```python
from build123d import *

# Parameters (mm, degrees)
BOSS_EXTRUDE1_DEPTH      = 40
BOSS_EXTRUDE1_DEPTH_BACK = 40
SKETCH2_W                = 140
SKETCH2_H                = 70
CUT_EXTRUDE1_DEPTH       = 16
SKETCH3_R                = 4
CUT_EXTRUDE2_DEPTH       = 5


with BuildPart() as part:
    # Sketch1 → Boss-Extrude1 (new, two sides: drawn at the far end of the back side and taken through both)
    with BuildSketch(Plane.XY.offset(-BOSS_EXTRUDE1_DEPTH_BACK)):
        with BuildLine():
            Line((-65, 10), (65, 10))
            ThreePointArc((65, 10), (75, 0), (65, -10))
            Line((65, -10), (-65, -10))
            ThreePointArc((-65, -10), (-75, 0), (-65, 10))
        make_face()
    extrude(amount=BOSS_EXTRUDE1_DEPTH + BOSS_EXTRUDE1_DEPTH_BACK)

    # Sketch2 → Cut-Extrude1 (cut)
    with BuildSketch(Plane(origin=(0, 10, 0), x_dir=(1, 0, 0), z_dir=(0, 1, 0))):
        Rectangle(SKETCH2_W, SKETCH2_H)
    extrude(amount=-CUT_EXTRUDE1_DEPTH, mode=Mode.SUBTRACT)

    # Sketch3 → Cut-Extrude2 (cut)
    with BuildSketch(Plane.XY.offset(40)):
        with Locations((65, 0)):
            Circle(SKETCH3_R)
        with Locations((-65, 0)):
            Circle(SKETCH3_R)
        with Locations((25, 0)):
            Circle(SKETCH3_R)
    extrude(amount=-CUT_EXTRUDE2_DEPTH, mode=Mode.SUBTRACT)


solid = part.part
```
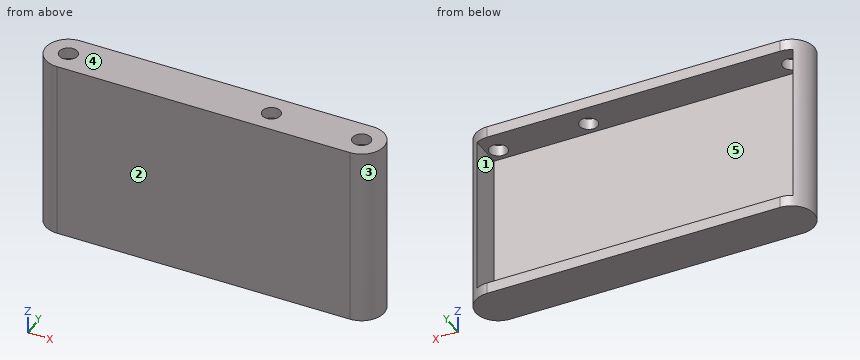
Design review of the part built by this model. Coordinates are the model's own, in mm. Face numbers are marked on the shaded views. A direction names the side the tool comes from. Give positions to 0.01 mm unless a question says otherwise; leave off trailing zeros. Order: outer loops, then holes, each group sorted by start corner. A loop starts at its lowest first (then second) coordinate and runs counter-clockwise, first axis right, second up. Notation, with made-up numbers: (67.5, -23.5) -> (121.5, -23.5) arc R23 cw to (121.5, 1.5) -> close; hole circle Ø11 at (57.5, 38.5). An arc over 180 degrees is marked (long way). Write each question's results on one line, items separated by ' | '. Start each with the question number.
Q1. Wall thickness on L1, parallel to Z at x = -44.5, y = -2.75; L2, parallel to Y at x = 25, z = 38.75; L3, parallel to Z at x = 65.5, y = -1.25: over which ranges is each line inside the solid? List them lowest first. Write a range as from..to.
Q2. Add section C-C on x = 51. Give the boundary of the cut face in (y, z), and give its area (3 significant figures).
Q3. Mouldability with a two-part tool opening along X and no side actions: class the marked faces 3, 4 and 5 as +X half, -X half, draft (parallel to the pull), parting line (faces both ways), or undercut.
Q4. Add section D-D on y = 6. Give the boundary of the cut face in (x, z), and give its area (3 significant figures).
Q5. Add section B-B on y = 0. Give the boundary of the cut face in (x, z).
Q6. For pin 1 (4.5 mm diameter, centred on y = 3.5, z = 10.5, fed in from +X); pin 2 (3 mm diameter, centred on y = 2, z = 12, fed in from +X); pin 3 (6 mm diameter, centred on x = 34, z = 24, fed in from +Y), all flat-tipped, find the tip position at first contact; note any pin that passes through.
Q7. Machinability: for the marked faces 1 and 2, which of the approach directions +Z, -Z, +X, -X, +Y, -Y give a long, thin tool a straight path to every point of the face, cutting with its end or side? Answer none if there is none.
Q8. Add section A-A on x = 25. Give the boundary of the cut face in (y, z).
Found:
1) L1: z = -40..-35, 35..40 | L2: y = -10..-4, 4..10 | L3: z = -40..-35
2) outline: (-10, -40) -> (10, -40) -> (10, -35) -> (-6, -35) -> (-6, 35) -> (10, 35) -> (10, 40) -> (-10, 40) -> close | area: 480 mm2
3) face 3: +X half | face 4: draft | face 5: undercut
4) outline: (-73, -40) -> (73, -40) -> (73, 40) -> (-73, 40) -> close; hole (-70, -35) -> (70, -35) -> (70, 35) -> (-70, 35) -> close | area: 1,880 mm2
5) outline: (-75, -40) -> (75, -40) -> (75, 40) -> (69, 40) -> (69, 35) -> (70, 35) -> (70, -35) -> (-70, -35) -> (-70, 35) -> (-69, 35) -> (-69, 40) -> (-75, 40) -> close; (-61, 35) -> (21, 35) -> (21, 40) -> (-61, 40) -> close; (29, 35) -> (61, 35) -> (61, 40) -> (29, 40) -> close
6) pin 1: stops at x = 74.92 | pin 2: stops at x = 74.99 | pin 3: stops at y = -6
7) face 1: +Y | face 2: +Z, -Z, +X, -X, -Y
8) outline: (-10, -40) -> (10, -40) -> (10, -35) -> (-6, -35) -> (-6, 35) -> (-4, 35) -> (-4, 40) -> (-10, 40) -> close; (4, 35) -> (10, 35) -> (10, 40) -> (4, 40) -> close
